```python
from build123d import *


with BuildPart() as part:
    # Sketch → Revolution (revolve)
    with BuildSketch(Plane.XY):
        with BuildLine():
            Line((43.25, 12.102886), (51.732051, 17))
            Line((51.732051, 17), (50, 20))
            Line((41.25, 14.948185), (50, 20))
            ThreePointArc((41.25, 14.948185), (36.49167, 10.189855), (34.75, 3.689855))
            Line((34.75, 3.689855), (34.75, -4))
            Line((34.75, -4), (37.75, -4))
            Line((37.75, 2.576606), (37.75, -4))
            ThreePointArc((43.25, 12.102886), (39.223721, 8.076606), (37.75, 2.576606))
        make_face()
    revolve(axis=Axis((0, 0, 0), (0, 1, 0)))


solid = part.part
```
Verification items for the finished model (mm, model axes). Give positions to 0.01 mm unless a question says otherwise; leave off trailing zeros. Order: outer loops, then holes, each group sorted by start corner. A loop starts at its lowest first (then second) coordinate and runs counter-clockwise, first axis right, second up. Notation, with made-up numbers: M -3.5,-7 L 3.5,-7 A26 ccw 3.5,24 Z; hole C -8,-33.5 d10. An arc over 180 degrees is marked long. Return JSON: item names as keys, results as strings. Group by question number.
1) Go/stop test with flat-tipped pins: pin 1 Ø12 at (x, z) = (-31.5, 16.5) entering from +Y; pin 2 Ø5 at (y, z) = (-1, -36.5) entering from +X; pin 3 Ø8 at (y, z) = (13, 27.5) entering from +X; pin 4 Ø10 at (x, z) = (30, -5) entering from -Y. Record where each tip stops, or that it passes through.
2) Section check D-D on y = 10.5. Record the cut outline in (x, z), and give its area (3 significant figures).
3) Section check A-A on x = 0. Record the cut outline in (y, z).
4) Mould release check, pull along Z, two halves, no side actions. Record for faces 1 (the face through (-5.441, 15.264, -41.442)), 2 (the face through (36.007, -0.758, -11.339)), 3 (the face through (-17, -4, 31)): pulls with the +Z half, pulls with the -Z half, needs draft (parallel to the pull), parting line crosses it, or undercut.
5) Scan lines: line 1 (X direction, y = 0.75, z = 0); line 2 (Z direction, x = 13.5, y = 7.5). Record each from-to range of solid material in increasing order.
6) Section check B-B on z = 0. Record the cut outline in (x, y), and give its area (3 significant figures).
7) Section check C-C on y = 1.25. Record the cut outline in (x, z), and give its area (3 significant figures).
Answer block:
{
 "1": {"pin 1": "stops at y = 15.13", "pin 2": "stops at x = 16.4", "pin 3": "stops at x = 44.18", "pin 4": "stops at y = -4"},
 "2": {"outline": "C 0,0 d82.24; hole C 0,0 d73.35", "area": "1,090 mm^2"},
 "3": {"outline": "M -4,-37.75 L 2.58,-37.75 A11 cw 12.1,-43.25 L 17,-51.73 L 20,-50 L 14.95,-41.25 A13 ccw 3.69,-34.75 L -4,-34.75 Z; M -4,34.75 L 3.69,34.75 A13 ccw 14.95,41.25 L 20,50 L 17,51.73 L 12.1,43.25 A11 cw 2.58,37.75 L -4,37.75 Z"},
 "4": {"face 1": "undercut", "face 2": "parting line crosses it", "face 3": "needs draft"},
 "5": {"line 1": "x = -37.75 to -34.75, 34.75 to 37.75", "line 2": "z = -36.5 to -32.64, 32.64 to 36.5"},
 "6": {"outline": "M -51.73,17 L -43.25,12.1 A11 cw -37.75,2.58 L -37.75,-4 L -34.75,-4 L -34.75,3.69 A13 ccw -41.25,14.95 L -50,20 Z; M 34.75,-4 L 37.75,-4 L 37.75,2.58 A11 cw 43.25,12.1 L 51.73,17 L 50,20 L 41.25,14.95 A13 ccw 34.75,3.69 Z", "area": "196 mm^2"},
 "7": {"outline": "C 0,0 d75.5; hole C 0,0 d69.5", "area": "683 mm^2"}
}
